Verification items for the finished model (mm, model axes). Give positions to 0.01 mm unless a question says otherwise; leave off trailing zeros. Loops run counter-clockwise (first coordinate to the right, second up) from the corner with the lowest first, then second, coordinate; pieces in that order, holes last. Notation, with made-up numbers: (64.25, 32) - (72.25, 32) arc R17 cw to (72.25, 37) - close; hole circle Ø1 at (47, 38.5). An arc over 180 degrees is marked (long way). One line per item, written item: value. Start each with the question number.
1. Sectioned sample at A-A (y = 0). Record the cut outline in (x, z), plus the area to 3 significant figures.
2. Sectioned sample at B-B (x = 106.5). Record the cut outline in (y, z), plus the area to 3 significant figures.
3. Gauge pin test, flat ends, axial feed: pin 1 (6.5 mm diameter, centred on y = 2, z = -2, fed in from -X); pin 2 (2 mm diameter, centred on x = 199, z = -5.5, fed in from -Y); pin 3 (10 mm diameter, centred on x = 294.5, y = 8, fed in from -Z); pin 4 (1.5 mm diameter, centred on y = -1, z = 7, fed in from -X). Record the tip position at first contact, or that the pin passes through.
4. Scan lines: L1, parallel to X at y = 0, z = 11.25; L2, parallel to Y at x = 540.5, z = 6.5; L3, parallel to Y at x = 611.5, z = -0.5. Record each from-to range of solid material in increasing order. Write a range as [from, to].
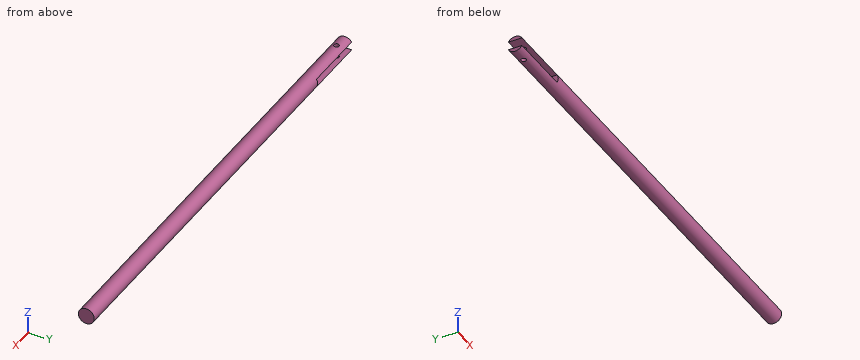
from build123d import *

# Parameters (mm, degrees)
F0_R          = 12.5
F1_DEPTH      = 735
F2_R          = 4
F3_DEPTH      = 12.5
F3_DEPTH_BACK = 12.5
F4_W          = 100
F4_H          = 13
F5_DEPTH      = 25.4
F5_DEPTH_BACK = 25.4


with BuildPart() as f1:
    # F0 (on Right) → F1 (new body)
    with BuildSketch(Plane.YZ):
        Circle(F0_R)
    extrude(amount=F1_DEPTH)

    # F2 (on Top) → F3 (cut, two sides)
    with BuildSketch(Plane.XY) as f3_sk:
        with Locations((24, 0)):
            Circle(F2_R)
    extrude(amount=-F3_DEPTH, mode=Mode.SUBTRACT)
    extrude(f3_sk.sketch, amount=F3_DEPTH_BACK, mode=Mode.SUBTRACT)

    # F4 (on Front) → F5 (cut, two sides)
    with BuildSketch(Plane.XZ) as f5_sk:
        with Locations((50, 0)):
            Rectangle(F4_W, F4_H)
    extrude(amount=-F5_DEPTH, mode=Mode.SUBTRACT)
    extrude(f5_sk.sketch, amount=F5_DEPTH_BACK, mode=Mode.SUBTRACT)


solid = f1.part
Results are:
1. outline: (0, -12.5) - (20, -12.5) - (20, -6.5) - (0, -6.5) - close; (0, 6.5) - (20, 6.5) - (20, 12.5) - (0, 12.5) - close; (28, -12.5) - (735, -12.5) - (735, 12.5) - (28, 12.5) - (28, 6.5) - (100, 6.5) - (100, -6.5) - (28, -6.5) - close
1. area: 17,000 mm^2
2. outline: circle Ø25 at (0, 0)
2. area: 491 mm^2
3. pin 1: stops at x = 100
3. pin 2: stops at y = -11.66
3. pin 3: stops at z = -12.13
3. pin 4: stops at x = 0
4. L1: x = [0, 20], [28, 735]
4. L2: y = [-10.68, 10.68]
4. L3: y = [-12.49, 12.49]
